For this review, use the dimensioned drawing (mm, ordinates from the lowest corner) and the shaded views. Coordinates: 2 decimals unless noted, no trailing zeros. Write each loop counter-clockwise with the first axis right and the second up, starting at its lowest first coordinate (ties: lowest second). Pieces come first, ordered by that corner, then holes.
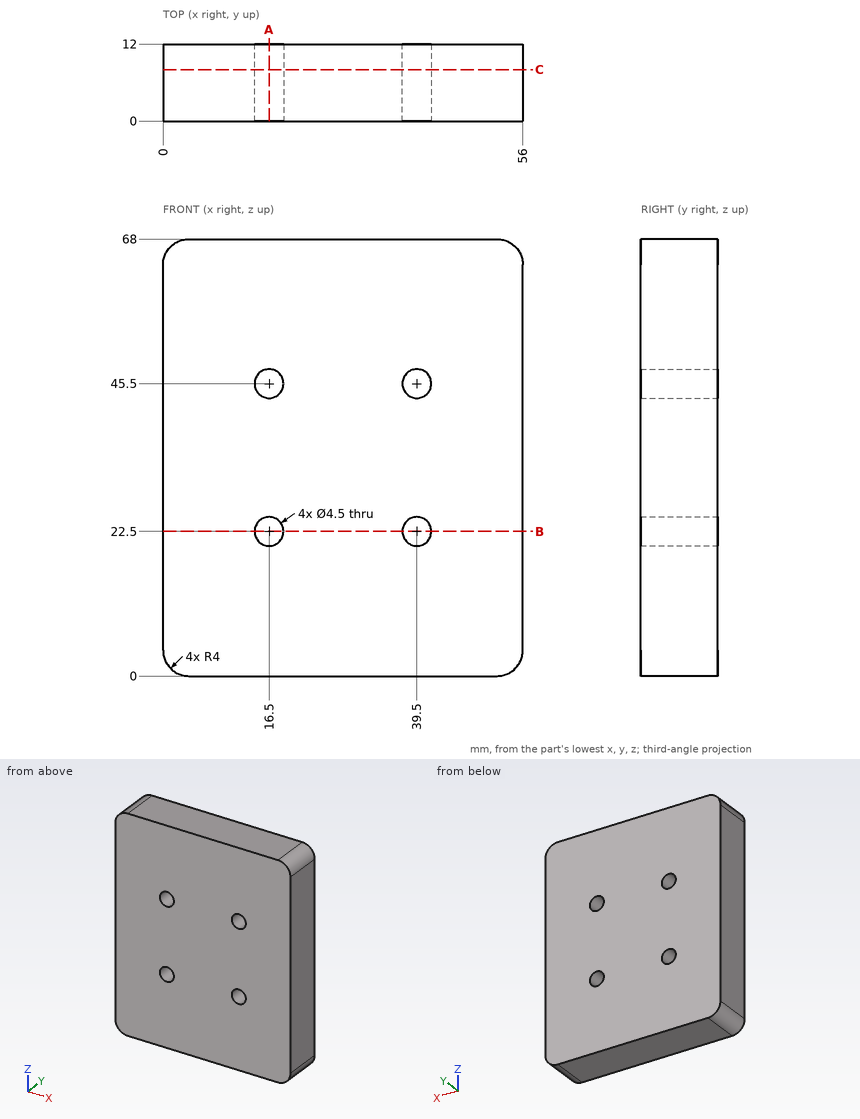
(1) Consider section A-A (x = 16.5). Give the boundary of the cut face in (y, z).
(2) Consider section C-C (y = 8). Give the boundary of the cut face in (x, z), plus the area to 3 significant figures.
(3) Wall thickness on line 1 (Z direction, x = 16.5, y = 9.5); line 2 (X direction, y = 7.5, z = 44): over which ranges is each line inside the solid? List them lowest first.
(4) Consider section B-B (z = 22.5). Give the boundary of the cut face in (x, y), plus the area to 3 significant figures.
(5) Insertion check: pin 1 Ø2.5 at (x, z) = (16.5, 45.5) entering from +Y. The pin has a flat end and moves straight along its axis. Give the tip position at first contact, or say it passes through.
Results:
1. outline: (0, 0) - (12, 0) - (12, 20.25) - (0, 20.25) - close; (0, 24.75) - (12, 24.75) - (12, 43.25) - (0, 43.25) - close; (0, 47.75) - (12, 47.75) - (12, 68) - (0, 68) - close
2. outline: (0, 4) arc R4 ccw to (4, 0) - (52, 0) arc R4 ccw to (56, 4) - (56, 64) arc R4 ccw to (52, 68) - (4, 68) arc R4 ccw to (0, 64) - close; hole circle Ø4.5 at (16.5, 22.5); hole circle Ø4.5 at (16.5, 45.5); hole circle Ø4.5 at (39.5, 22.5); hole circle Ø4.5 at (39.5, 45.5)
2. area: 3,730 mm2
3. line 1: z = 0 to 20.25, 24.75 to 43.25, 47.75 to 68
3. line 2: x = 0 to 14.82, 18.18 to 37.82, 41.18 to 56
4. outline: (0, 0) - (14.25, 0) - (14.25, 12) - (0, 12) - close; (18.75, 0) - (37.25, 0) - (37.25, 12) - (18.75, 12) - close; (41.75, 0) - (56, 0) - (56, 12) - (41.75, 12) - close
4. area: 564 mm2
5. pin 1: passes through
